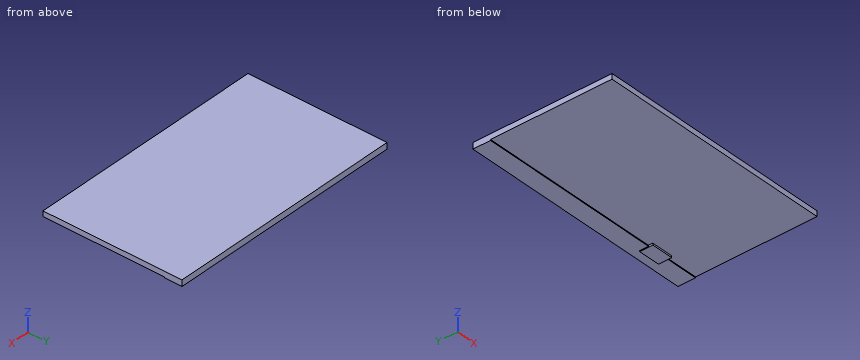
from build123d import *

# Parameters (mm, degrees)
ESQUISSE1_W        = 545
ESQUISSE1_H        = 318
BOSS_EXTRU_1_DEPTH = 12
ESQUISSE2_W        = 545
ESQUISSE2_H        = 40
BOSS_EXTRU_2_DEPTH = 2
ESQUISSE3_W        = 50
ESQUISSE3_H        = 30
BOSS_EXTRU_3_DEPTH = 4


with BuildPart() as part:
    # Esquisse1 → Boss.-Extru.1 (new body)
    with BuildSketch(Plane.XY):
        Rectangle(ESQUISSE1_W, ESQUISSE1_H)
    extrude(amount=BOSS_EXTRU_1_DEPTH)

    # Esquisse2 → Boss.-Extru.2 (add)
    with BuildSketch(Plane(origin=(0, 0, 0), x_dir=(-1, 0, 0), z_dir=(0, 0, -1))):
        with Locations((0, 139)):
            Rectangle(ESQUISSE2_W, ESQUISSE2_H)
    extrude(amount=BOSS_EXTRU_2_DEPTH)

    # Esquisse3 → Boss.-Extru.3 (add)
    with BuildSketch(Plane(origin=(0, 0, 0), x_dir=(-1, 0, 0), z_dir=(0, 0, -1))):
        with Locations((-172.5, 124)):
            Rectangle(ESQUISSE3_W, ESQUISSE3_H)
    extrude(amount=BOSS_EXTRU_3_DEPTH)


solid = part.part
The model under review builds one solid part; all positions refer to its coordinate system, in mm. Round coordinates to 2 decimals unless told otherwise and drop trailing zeros. Loops run counter-clockwise (first coordinate to the right, second up) from the corner with the lowest first, then second, coordinate; pieces in that order, holes last. Notation, with made-up numbers: M -7,76 L 44,76 A16 cw 44,102 Z; hole C -24.5,-11.5 d8. An arc over 180 degrees is marked long. Answer as a JSON object with one key per item and string values.
Item 1: Clearance check with flat-ended pins moving along their axes: P1, Ø4, axis at x = 111, y = 55, coming from the -Z side; P2, Ø0.6, axis at x = 184, z = -3, coming from the +Y side; P3, Ø12, axis at x = -94, y = 139, coming from the -Z side. State where each tip first meets the part, or that it passes through.
Check sheet entries:
{"P1": "z = 0", "P2": "y = 139", "P3": "z = -2"}
Item 2: For line 1 along Z through (x, y) = (-188, 0); line 2 along Y through (x, z) = (140.5, -1), list the stretches that pass through material, from the lowest coordinate up.
Check sheet entries:
{"line 1": "0 to 12", "line 2": "119 to 159"}
Item 3: We need section C-C, the plane x = 181. State the section outline as (y, z) points, and give its area (3 significant figures).
Check sheet entries:
{"outline": "M -159,0 L 109,0 L 109,-4 L 139,-4 L 139,-2 L 159,-2 L 159,12 L -159,12 Z", "area": "3,980 mm2"}
Item 4: We need section B-B, the plane x = -25.5. State the section outline as (y, z) points, and give its area (3 significant figures).
Check sheet entries:
{"outline": "M -159,0 L 119,0 L 119,-2 L 159,-2 L 159,12 L -159,12 Z", "area": "3,900 mm2"}
Item 5: We need section A-A, the plane y = 124.5. State the section outline as (x, z) points.
Check sheet entries:
{"outline": "M -272.5,-2 L 147.5,-2 L 147.5,-4 L 197.5,-4 L 197.5,-2 L 272.5,-2 L 272.5,12 L -272.5,12 Z"}
